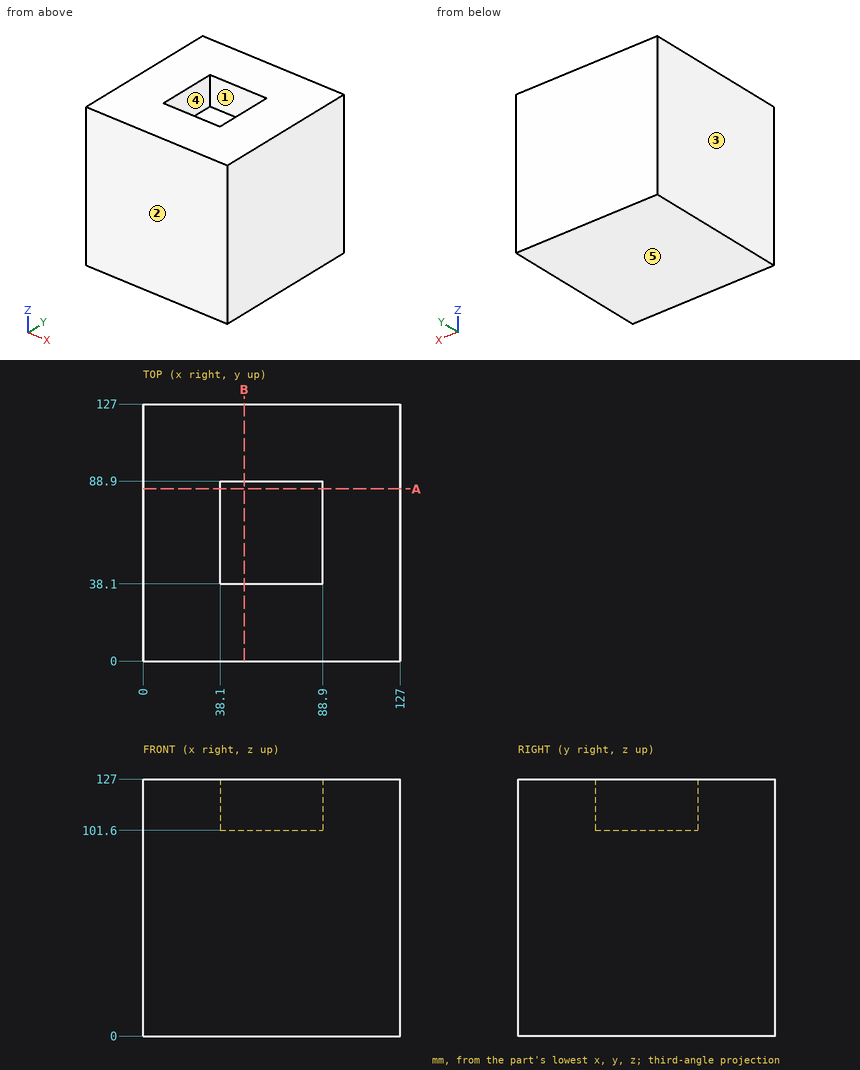
The drawing under review shows one solid part. Ordinate dimensions are in mm from its lowest x, y, z. A direction names the side the tool comes from. Round coordinates to 2 decimals unless told otherwise and drop trailing zeros. Write each loop counter-clockwise with the first axis right and the second up, starting at its lowest first coordinate (ties: lowest second). Pieces come first, ordered by that corner, then holes.
(1) We need section A-A on y = 85. Give the boundary of the cut face in (x, z), and give its area (3 significant figures).
(2) Insertion check: pin 1 (12.5 mm diameter, centred on y = 53, z = 119.5, fed in from -X). The pin has a flat end and moves straight along its axis. Give the tip position at first contact, or say it passes through.
(3) Wall thickness on L1, parallel to X at y = 59, z = 111; L2, parallel to Z at x = 49, y = 42.5: over which ranges is each line inside the solid? List them lowest first.
(4) Machinability: for the marked faces 4 and 5, which of the approach directions +Z, -Z, +X, -X, +Y, -Y give a long, thin tool a straight path to every point of the face, cutting with its end or side? Answer none if there is none.
(5) Mouldability with a two-part tool opening along X and no side actions: class the marked faces 1, 2 and 3 as +X half, -X half, draft (parallel to the pull), parting line (faces both ways), or undercut.
Findings below:
1. outline: (0, 0) - (127, 0) - (127, 127) - (88.9, 127) - (88.9, 101.6) - (38.1, 101.6) - (38.1, 127) - (0, 127) - close
1. area: 14,800 mm2
2. pin 1: stops at x = 0
3. L1: x = 0 to 38.1, 88.9 to 127
3. L2: z = 0 to 101.6
4. face 4: +Z
4. face 5: -Z, +X, -X, +Y, -Y
5. face 1: undercut
5. face 2: draft
5. face 3: -X half
